Read the model definition and answer for the solid it produces. Units are mm, in the model's axes. Round coordinates to 2 decimals unless told otherwise and drop trailing zeros. Write each loop counter-clockwise with the first axis right and the second up, starting at its lowest first coordinate (ties: lowest second). Pieces come first, ordered by that corner, then holes. Notation, with made-up numbers: (-40, 47) - (6, 47) arc R15 ccw to (6, 61) - close; hole circle Ø2 at (69, 17.5). An arc over 180 degrees is marked (long way). One line per item, written item: value. Start each with the question number.
(1) Find the intervals of material crossed by L1, parallel to Y at x = 50.8, z = 4.5; L2, parallel to Y at x = 65, z = 6; L3, parallel to Y at x = 25.4, z = 5, in increasing order.
(2) Flat-ended cylindrical pins translate along their axes: pin 1 Ø3 at (x, z) = (107, 5) entering from +Y; pin 2 Ø2 at (y, z) = (42, 2) entering from +X. Find the tip coordinate at first contact, or state that the pin passes through.
(3) A cutting plane is placed at A-A, the plane x = 63.5. Determine the outline of the cut face in (y, z), plus the area to 3 significant figures.
(4) The mould has two halves that part along Y. Classify faces 1 (the face through (125.09, 1.81, 3.22)), 2 (the face through (127, 21, 3)), 3 (the face through (66.05, 12.81, 3.13)): +Y half, -Y half, draft (parallel to the pull), parting line (faces both ways), or undercut.
(5) A cutting plane is placed at B-B, the plane z = 3.5. State how many separate pieces and enclosed holes the cut face has, plus the area to 3 significant figures.
(6) A cutting plane is placed at C-C, the plane x = 12.7. Determine the outline of the cut face in (y, z), plus the area to 3 significant figures.
from build123d import *

# Parameters (mm, degrees)
SKETCH1_W               = 127
SKETCH1_H               = 82.55
BOSS_EXTRUDE1_DEPTH     = 6.35
SKETCH2_R               = 2.5527
CUT_EXTRUDE1_DEPTH      = 1
CUT_EXTRUDE1_DEPTH_BACK = 7.35
SKETCH3_R               = 2.4892
SKETCH3_R_2             = 2.5527
CUT_EXTRUDE2_DEPTH      = 7.35
CUT_EXTRUDE3_DEPTH      = 7.35
CUT_EXTRUDE4_DEPTH      = 7.35
FILLET1_R               = 6.35


with BuildPart() as part:
    # Sketch1 → Boss-Extrude1 (new body)
    with BuildSketch(Plane.XY):
        with Locations((63.5, 41.275)):
            Rectangle(SKETCH1_W, SKETCH1_H)
    extrude(amount=BOSS_EXTRUDE1_DEPTH)

    # Sketch2 → Cut-Extrude1 (cut, two sides)
    with BuildSketch(Plane(origin=(0, 0, 0), x_dir=(-1, 0, 0), z_dir=(0, 0, -1))) as cut_extrude1_sk:
        with Locations((-76.2, 63.5)):
            Circle(SKETCH2_R)
        with Locations((-63.5, 63.5)):
            Circle(SKETCH2_R)
        with Locations((-50.8, 63.5)):
            Circle(SKETCH2_R)
    extrude(amount=CUT_EXTRUDE1_DEPTH, mode=Mode.SUBTRACT)
    extrude(cut_extrude1_sk.sketch, amount=-CUT_EXTRUDE1_DEPTH_BACK, mode=Mode.SUBTRACT)

    # Sketch3 → Cut-Extrude2 (cut, through all)
    with BuildSketch(Plane(origin=(0, 0, 0), x_dir=(-1, 0, 0), z_dir=(0, 0, -1))):
        with Locations((-114.3, 38.1)):
            Circle(SKETCH3_R)
        with Locations((-114.3, 12.7)):
            Circle(SKETCH3_R_2)
        with Locations((-101.6, 38.1)):
            Circle(SKETCH3_R)
        with Locations((-101.6, 12.7)):
            Circle(SKETCH3_R_2)
        with Locations((-88.9, 38.1)):
            Circle(SKETCH3_R)
        with Locations((-88.9, 12.7)):
            Circle(SKETCH3_R_2)
        with Locations((-76.2, 38.1)):
            Circle(SKETCH3_R)
        with Locations((-76.2, 12.7)):
            Circle(SKETCH3_R_2)
        with Locations((-63.5, 38.1)):
            Circle(SKETCH3_R)
        with Locations((-63.5, 12.7)):
            Circle(SKETCH3_R_2)
        with Locations((-50.8, 38.1)):
            Circle(SKETCH3_R)
        with Locations((-50.8, 12.7)):
            Circle(SKETCH3_R_2)
        with Locations((-38.1, 38.1)):
            Circle(SKETCH3_R)
        with Locations((-38.1, 12.7)):
            Circle(SKETCH3_R_2)
        with Locations((-25.4, 38.1)):
            Circle(SKETCH3_R)
        with Locations((-25.4, 12.7)):
            Circle(SKETCH3_R_2)
        with Locations((-12.7, 38.1)):
            Circle(SKETCH3_R)
        with Locations((-12.7, 12.7)):
            Circle(SKETCH3_R_2)
    extrude(amount=-CUT_EXTRUDE2_DEPTH, mode=Mode.SUBTRACT)

    # Sketch4 → Cut-Extrude3 (cut, through all)
    with BuildSketch(Plane(origin=(0, 0, 0), x_dir=(-1, 0, 0), z_dir=(0, 0, -1))):
        Polygon((-83.82, 82.55), (-127, 39.37), (-127, 82.55), align=None)
        Polygon((-43.18, 82.55), (0, 82.55), (0, 39.37), align=None)
    extrude(amount=-CUT_EXTRUDE3_DEPTH, mode=Mode.SUBTRACT)

    # Sketch5 → Cut-Extrude4 (cut, through all)
    with BuildSketch(Plane(origin=(0, 0, 0), x_dir=(-1, 0, 0), z_dir=(0, 0, -1))):
        Polygon((-90.17, 76.2), (-36.83, 76.2), (-43.18, 82.55), (-83.82, 82.55), align=None)
    extrude(amount=-CUT_EXTRUDE4_DEPTH, mode=Mode.SUBTRACT)

    # Fillet1
    fillet1_edges = [part.edges().sort_by_distance(p)[0] for p in [
        (127, 39.37, 3.175),
        (0, 39.37, 3.175),
        (90.17, 76.2, 3.175),
        (36.83, 76.2, 3.175),
        (127, 0, 3.175),
        (0, 0, 3.175),
    ]]
    fillet(fillet1_edges, radius=FILLET1_R)


solid = part.part
Here are the results:
1. L1: 0 to 10.15, 15.25 to 35.61, 40.59 to 60.95, 66.05 to 76.2
1. L2: 0 to 10.63, 14.77 to 36.11, 40.09 to 61.43, 65.57 to 76.2
1. L3: 0 to 10.15, 15.25 to 35.61, 40.59 to 64.77
2. pin 1: y = 60.87
2. pin 2: x = 125.36
3. outline: (0, 0) - (10.15, 0) - (10.15, 6.35) - (0, 6.35) - close; (15.25, 0) - (35.61, 0) - (35.61, 6.35) - (15.25, 6.35) - close; (40.59, 0) - (60.95, 0) - (60.95, 6.35) - (40.59, 6.35) - close; (66.05, 0) - (76.2, 0) - (76.2, 6.35) - (66.05, 6.35) - close
3. area: 387 mm²
4. face 1: -Y half
4. face 2: draft
4. face 3: undercut
5. separate pieces: 1
5. enclosed holes: 21
5. area: 7,880 mm²
6. outline: (0, 0) - (10.15, 0) - (10.15, 6.35) - (0, 6.35) - close; (15.25, 0) - (35.61, 0) - (35.61, 6.35) - (15.25, 6.35) - close; (40.59, 0) - (52.07, 0) - (52.07, 6.35) - (40.59, 6.35) - close
6. area: 267 mm²
